Read the model definition and answer for the solid it produces. Units are mm, in the model's axes. Face numbers are marked on the shaded views. Round coordinates to 2 decimals unless told otherwise and drop trailing zeros. Order: outer loops, then holes, each group sorted by start corner. A loop starts at its lowest first (then second) coordinate and runs counter-clockwise, first axis right, second up. Notation, with made-up numbers: (1.25, 50) -> (7.25, 50) arc R25 cw to (7.25, 88) -> close; hole circle Ø4 at (54, 33). An arc over 180 degrees is marked (long way). Answer as a JSON object with one key per item and string values. Group by question number.
Item 1: Section D-D, the plane x = 4 is taken. Write down the section's boundary in (y, z).
Item 2: Section A-A, the plane z = 0 is taken. Write down the section's boundary in (x, y).
Item 3: Given P1, Ø12, axis at y = -4, z = 4, coming from the -X side, flat-ended and moving along its own axis, determine where the tip first touches the part or whether it passes through.
Item 4: The mould has two halves that part along Y. Classify the marked faces 1, 2 and 3: pulls with the +Y half, pulls with the -Y half, needs draft (parallel to the pull), parting line crosses it, or undercut.
Item 5: Section B-B, the plane x = 2 is taken. Write down the section's boundary in (y, z), plus the area to 3 significant figures.
Item 6: Consider probe 1 along Z at (x, y) = (5.75, 2); probe 2 along Y at (x, z) = (6, -2); probe 3 along Z at (x, y) = (4, 0.5). Determine where each line is inside the solid, lowest interval first. Write a range as from..to.
Item 7: Section C-C, the plane y = 1.5 is taken. Count the separate pieces of the cut face and the enclosed holes in it, plus the area to 3 significant figures.
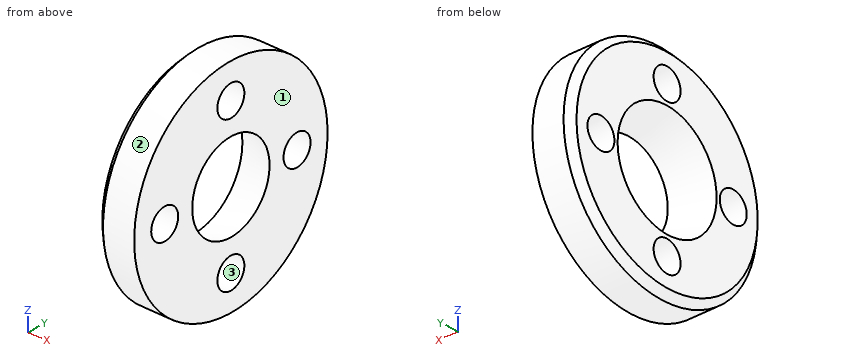
Autodesk Inventor part; units mm, degrees
ref_plane "at2_gew_st_XY" through (6.65, 0, 0) normal (1, 0, 0) x (0, 0, -1)
ref_plane "at2_gew_st_YZ" through (6.65, 0, 0) normal (0, 0, -1) x (0, 1, 0)
ref_plane "at2_gew_st_ZX" through (6.65, 0, 0) normal (0, 1, 0) x (1, 0, 0)
sketch "Sketch_7" plane through (0, 0, 0) normal (0, 0, 1) x (1, 0, 0)
  line L0 (6.65, 0) -> (0, 0)
  line L1 (0, 0) -> (0, 17.8)
  line L2 (0, 17.8) -> (1.2, 19)
  line L3 (1.2, 19) -> (6.65, 19)
  line L4 (6.65, 19) -> (6.65, 0)
  line L5 (6.65, 0) -> (0, 0)
revolve "Revolution1" add sketch "Sketch_7" angle 360 about axis through (6.65, 0, 0) along (1, 0, 0)
sketch "Sketch_8" plane through (0, 0, 0) normal (0, 0, 1) x (1, 0, 0)
  line L0 (6.65, 0) -> (0, 0)
  line L1 (0, 0) -> (0, 9.728)
  line L2 (0, 9.728) -> (6.65, 7.6)
  line L3 (6.65, 7.6) -> (6.65, 0)
  line L4 (6.65, 0) -> (0, 0)
revolve "Revolution2" cut sketch "Sketch_8" angle 360 about axis through (6.65, 0, 0) along (1, 0, 0)
sketch "Sketch3" plane through (6.65, 0, 0) normal (1, 0, 0) x (0, 0, -1)
  point P0 (0, 13)
hole "Hole1" at (6.65, 13, 0) direction (-1, 0, 0) diameter 5.3 depth 6.65
pattern_linear "Rectangular Pattern1" count 2 spacing 18.3848 along (0, -0.7071, 0.7071) count 2 spacing 18.3848 along (0, -0.7071, -0.7071) of "Hole1"
ref_plane "at2_gew_st_XY" through (6.65, 0, 0) normal (1, 0, 0) x (0, 0, -1)
ref_plane "at2_gew_st_YZ" through (6.65, 0, 0) normal (0, 0, -1) x (0, 1, 0)
ref_plane "at2_gew_st_ZX" through (6.65, 0, 0) normal (0, 1, 0) x (1, 0, 0)
ref_plane "schr_1_XY" through (6.65, 13, 0) normal (1, 0, 0) x (0, 0, -1)
ref_plane "schr_1_YZ" through (6.65, 13, 0) normal (0, 0, -1) x (0, 1, 0)
ref_plane "schr_1_ZX" through (6.65, 13, 0) normal (0, 1, 0) x (1, 0, 0)
ref_plane "schr_2_XY" through (6.65, 0, -13) normal (1, 0, 0) x (0, 0, -1)
ref_plane "schr_2_YZ" through (6.65, 0, -13) normal (0, 0, -1) x (0, 1, 0)
ref_plane "schr_2_ZX" through (6.65, 0, -13) normal (0, 1, 0) x (1, 0, 0)
ref_plane "schr_3_XY" through (6.65, -13, 0) normal (1, 0, 0) x (0, 0, -1)
ref_plane "schr_3_YZ" through (6.65, -13, 0) normal (0, 0, -1) x (0, 1, 0)
ref_plane "schr_3_ZX" through (6.65, -13, 0) normal (0, 1, 0) x (1, 0, 0)
ref_plane "schr_4_XY" through (6.65, 0, 13) normal (1, 0, 0) x (0, 0, -1)
ref_plane "schr_4_YZ" through (6.65, 0, 13) normal (0, 0, -1) x (0, 1, 0)
ref_plane "schr_4_ZX" through (6.65, 0, 13) normal (0, 1, 0) x (1, 0, 0)
properties part number "61581400_4"
Values found:
{
 "1": {"outline": "circle Ø38 at (0, 0); hole circle Ø5.3 at (-13, 0); hole circle Ø16.9 at (0, 0); hole circle Ø5.3 at (0, -13); hole circle Ø5.3 at (0, 13); hole circle Ø5.3 at (13, 0)"},
 "2": {"outline": "(0, -17.8) -> (1.2, -19) -> (6.65, -19) -> (6.65, -15.65) -> (0, -15.65) -> close; (0, -10.35) -> (6.65, -10.35) -> (6.65, -7.6) -> (0, -9.73) -> close; (0, 9.73) -> (6.65, 7.6) -> (6.65, 10.35) -> (0, 10.35) -> close; (0, 15.65) -> (6.65, 15.65) -> (6.65, 19) -> (1.2, 19) -> (0, 17.8) -> close"},
 "3": {"P1": "x = 0"},
 "4": {"face 1": "needs draft", "face 2": "parting line crosses it", "face 3": "undercut"},
 "5": {"outline": "circle Ø38 at (0, 0); hole circle Ø5.3 at (-13, 0); hole circle Ø18.18 at (0, 0); hole circle Ø5.3 at (0, -13); hole circle Ø5.3 at (0, 13); hole circle Ø5.3 at (13, 0)", "area": "786 mm2"},
 "6": {"probe 1": "-18.89..-14.74, -11.26..-7.63, 7.63..11.26, 14.74..18.89", "probe 2": "-18.89..-14.74, -11.26..-7.55, 7.55..11.26, 14.74..18.89", "probe 3": "-18.99..-15.6, -10.4..-8.43, 8.43..10.4, 15.6..18.99"},
 "7": {"separate pieces": "4", "enclosed holes": "0", "area": "78.9 mm2"}
}
